from build123d import *

# Parameters (mm, degrees)
F0_W      = 50
F0_H      = 12.5
F1_DEPTH  = 8
F2_DEPTH  = 75
F4_DEPTH  = 8
F7_DEPTH  = 3
F8_DEPTH  = 1
F11_DEPTH = 3
F14_DEPTH = 3
F15_DEPTH = 8
F16_DEPTH = 8


# Not quite as in the source:
# - a feature names something its author has since deleted; it is built from what else it names


with BuildPart() as f1:
    # F0 (on Top) → F1 (new body)
    with BuildSketch(Plane.XY):
        Polygon((57.9695070384, 39.3207329262), (60.5095952989, 40.7487522591), (42.0179491924, 72.7772228311), (-42.0179491924, 72.7772228311), (-84.0358983849, 0), (-42.0179491924, -72.7772228311), (42.0179491924, -72.7772228311), (84.0358983849, 0), (65.5097997054, 32.0881441788), (62.870004896, 30.6039762231), (65.3204122546, 26.2455930623), (60.0654171506, 23.2910848888), (57.615009792, 27.6494680496), (55.164720758, 32.0079177338), (52.7144317239, 36.366367418), (50.2642610162, 40.7248836223), (55.5194165334, 43.6791064608), align=None)
        with Locations((0, 54.5829171234)):
            Rectangle(F0_W, F0_H, mode=Mode.SUBTRACT)
    extrude(amount=F1_DEPTH)

    # F0 (on Top) → F2 (join)
    with BuildSketch(Plane.XY):
        Polygon((-84.0358983849, 0), (-87.5, 0), (-68.1246734519, -33.5590499945), (-63.1251610364, -42.2184595112), (-43.75, -75.7772228311), (43.75, -75.7772228311), (87.5, 0), (84.0358983849, 0), (42.0179491924, -72.7772228311), (-42.0179491924, -72.7772228311), align=None)
    extrude(amount=F2_DEPTH)

    # F0 (on Top) → F4 (join)
    with BuildSketch(Plane.XY):
        Polygon((43.75, 75.7772228311), (-43.75, 75.7772228311), (-65.625, 37.8886114156), (-68.125, 33.5584843966), (-87.5, 0), (-84.0358983849, 0), (-42.0179491924, 72.7772228311), (42.0179491924, 72.7772228311), (60.5095952989, 40.7487522591), (63.1248363216, 42.2190219338), align=None)
    extrude(amount=F4_DEPTH)

    # F6 (on face) → F7 (join)
    with BuildSketch(Plane(origin=(0, -50.1312366318, 89.3836679776), x_dir=(1, 0, 0), z_dir=(0, 0.4891706574, -0.872188092))):
        Polygon((43.75, 29.4041920927), (0, 29.4041920927), (-43.75, 29.4041920927), (-42.01795, -57.4775522498), (42.01795, -57.4775522498), align=None)
    extrude(amount=F7_DEPTH)

    # F3 (on Front) → F8 (join)
    with BuildSketch(Plane.XZ):
        Polygon((-42.01795, 114.5), (0, 114.5), (42.01795, 114.5), (84.0359, 75), (87.5, 75), (42.01795, 117.5), (0, 117.5), (-42.01795, 117.5), (-87.5, 75), (-84.0359, 75), align=None)
    extrude(amount=F8_DEPTH)

    # F10 (on face) → F11 (join)
    with BuildSketch(Plane(origin=(-67.6846727043, -39.0777640058, 72.4338274863), x_dir=(0.7723629594, -0.3015876344, 0.5590173143), z_dir=(-0.6351814378, -0.3667221741, 0.6797495039))):
        Polygon((33.2314262259, 55.789645187), (-25.6554603702, 35.6104118215), (30.9888924807, -31.0804218073), align=None)
    extrude(amount=-F11_DEPTH)

    # F13 (on face) → F14 (join)
    with BuildSketch(Plane(origin=(67.6756688636, -39.5950852503, 72.4241918832), x_dir=(0.7733047167, 0.3041472681, -0.556322078), z_dir=(-0.6340345536, 0.3709553614, -0.6785221475))):
        Polygon((-30.939509805, 30.5117392321), (-32.8751652468, -56.3649154418), (25.9400068576, -35.9776056011), align=None)
    extrude(amount=F14_DEPTH)

    # F0 (on Top) → F15 (join)
    with BuildSketch(Plane.XY):
        with Locations((0, 54.5829171234)):
            Rectangle(F0_W, F0_H)
    extrude(amount=F15_DEPTH)

    # F0 (on Top) → F16 (join)
    with BuildSketch(Plane.XY):
        Polygon((-77.8456264388, -39.3203929827), (-73.5443198074, -36.7711261738), (-75.8386599429, -32.8999502926), (-80.1399666105, -35.4492170403), align=None)
        Polygon((-63.1251610364, -42.2184595112), (-68.1246734519, -33.5590499945), (-73.5443198074, -36.7711261738), (-77.8456264388, -39.3203929827), (-72.8456167613, -47.9806414332), (-68.5445301574, -45.4310034146), align=None)
        Polygon((-66.2498559406, -49.3019813581), (-68.5445301574, -45.4310034146), (-72.8456167613, -47.9806414332), (-70.5509425445, -51.8516193767), align=None)
    extrude(amount=F16_DEPTH)


solid = f1.part
Design review of the part built by this model. Coordinates are the model's own, in mm. A direction names the side the tool comes from. Round coordinates to 2 decimals unless told otherwise and drop trailing zeros. Write each loop counter-clockwise with the first axis right and the second up, starting at its lowest first coordinate (ties: lowest second). Pieces come first, ordered by that corner, then holes. Notation, with made-up numbers: M 40.25,13.5 L 63.25,13.5 A18 cw 63.25,38.5 Z; hole C 89.5,55.5 d5. An arc over 180 degrees is marked long. One line per item, written item: value. Start each with the question number.
1. Take a section at A-A on z = 24. State the section outline as (x, y) points, then the cut area to 3 significant figures.
2. Draft analysis for pull direction Z (two halves, no side actions). For faces 4 (the face through (63.32, -35.88, 40.72)), 5 (the face through (-54.822, -24.821, 92.145)), 6 (the face through (1, 75.777, 4)), state which applies: pulls with the +Z half, pulls with the -Z half, needs draft (parallel to the pull), parting line crosses it, or undercut.
3. To check wall thickness, follow probe 1 along X at (y, z) = (-34, 49.5); probe 2 along Y at (x, z) = (15, 40.5); probe 3 along Z at (x, y) = (-45, 27). State the ranges of each line that lie inside material, in increasing order. Write a range as from..to.
4. Take a section at C-C on y = -7. State the section outline as (x, z) points.
5. For faces 1 (the face through (-0.612, -38.912, 95.676)), 2 (the face through (56.727, 41.53, 3.944)), 3 (the face through (-53.7, -22, 90.3)), list the 3-axis set-ups (+Z, -Z, +X, -X, +Y, -Y) from which the entire face can be reached by the end or side of a thin tool; tool diameter is ignored.
6. Take a section at B-B on x = 9.5. State the section outline as (y, z) points.
7. Clearance check with flat-ended pins moving along their axes: P1, Ø8.5, axis at x = -75, y = -39.5, coming from the +Z side; P2, Ø1.7, axis at x = 86, z = 43, coming from the +Y side; P3, Ø2, axis at y = -28, z = 73.5, coming from the +X side. State where each tip first meets the part, or that it passes through.
8. Take a section at D-D on y = -61. State the section outline as (x, z) points, then the cut area to 3 significant figures.
Computed:
1. outline: M -87.5,0 L -43.75,-75.78 L 43.75,-75.78 L 87.5,0 L 84.04,0 L 42.02,-72.78 L -42.02,-72.78 L -84.04,0 Z
1. area: 772 mm²
2. face 4: undercut
2. face 5: pulls with the +Z half
2. face 6: needs draft
3. probe 1: x = -67.87..-64.41, 64.41..67.87
3. probe 2: y = -75.78..-72.78
3. probe 3: z = 0..8
4. outline: M -83.46,0 L 83.46,0 L 83.46,75 L 83.74,75.23 L 42.39,113.87 L 42.18,113.57 L -42.18,113.57 L -83.46,75 Z; hole M -79.99,8 L 79.99,8 L 79.99,74.31 L 41.66,110.13 L -41.14,110.13 L -79.99,73.82 Z
5. face 1: +Z, -X, -Y
5. face 2: +Z, -Z
5. face 3: +Y
6. outline: M -75.78,0 L 75.78,0 L 75.78,8 L -72.78,8 L -72.78,73.24 L 1.47,114.88 L 0,117.5 L -1,117.5 L -1,116.94 L -75.78,75 Z
7. P1: stops at z = 8
7. P2: stops at y = 0
7. P3: stops at x = 71.91
8. outline: M -52.28,0 L 52.28,0 L 52.28,75 L 52.34,75.05 L 43.46,83.35 L 43.41,83.29 L -43.41,83.29 L -52.28,75 Z; hole M -48.82,8 L 48.82,8 L 48.82,73.92 L 42.48,79.85 L -42.37,79.85 L -48.82,73.82 Z
8. area: 1,660 mm²
